from build123d import *

# Parameters (mm, degrees)
BOSS_EXTRUDE1_DEPTH = 10
FILLET1_R           = 1
FILLET2_R           = 0.5
FILLET3_R           = 1


with BuildPart() as part:
    # Sketch1 → Boss-Extrude1 (new body)
    with BuildSketch(Plane.XY):
        with BuildLine():
            Line((0.05, 14.37), (0.05, 3.706076092))
            ThreePointArc((0.05, 3.706076092), (1.009905384, 4.156578123), (2.05, 4.362911872))
            Line((2.05, 4.362911872), (2.05, 14.37))
            ThreePointArc((2.05, 14.37), (0.989726548, 16.929726548), (-1.57, 17.99))
            Line((-1.57, 17.99), (-2.748, 17.99))
            ThreePointArc((-2.748, 17.99), (-5.307726548, 16.929726548), (-6.368, 14.37))
            Line((-6.368, 14.37), (-4.368, 14.37))
            ThreePointArc((-4.368, 14.37), (-3.893512986, 15.515512986), (-2.748, 15.99))
            Line((-2.748, 15.99), (-1.57, 15.99))
            ThreePointArc((-1.57, 15.99), (-0.424487014, 15.515512986), (0.05, 14.37))
        make_face()
        with BuildLine():
            Line((0.05, -0.484767986), (0.05, -3.706076092))
            ThreePointArc((0.05, -3.706076092), (1.009905384, -4.156578123), (2.05, -4.362911872))
            Line((2.05, -4.362911872), (2.05, -2.352658071))
            ThreePointArc((2.05, -2.352658071), (0.753926793, -1.73572655), (0.05, -0.484767986))
        make_face()
        with BuildLine():
            ThreePointArc((2.05, 4.362911872), (1.009905384, 4.156578123), (0.05, 3.706076092))
            Line((0.05, 3.706076092), (0.05, 0.484767986))
            ThreePointArc((0.05, 0.484767986), (0.753926793, 1.73572655), (2.05, 2.352658071))
            Line((2.05, 2.352658071), (2.05, 4.362911872))
        make_face()
        with BuildLine():
            Line((2.05, -2.352658071), (2.05, -4.362911872))
            ThreePointArc((2.05, -4.362911872), (5.351470225, -3.206438835), (6.75, 0))
            ThreePointArc((6.75, 0), (5.351470225, 3.206438835), (2.05, 4.362911872))
            Line((2.05, 4.362911872), (2.05, 2.352658071))
            ThreePointArc((2.05, 2.352658071), (3.935248378, 1.790600458), (4.75, 0))
            ThreePointArc((4.75, 0), (3.935248378, -1.790600458), (2.05, -2.352658071))
        make_face()
        with BuildLine():
            Line((-1.57, -15.99), (-2.748, -15.99))
            ThreePointArc((-2.748, -15.99), (-3.893512986, -15.515512986), (-4.368, -14.37))
            Line((-4.368, -14.37), (-6.368, -14.37))
            ThreePointArc((-6.368, -14.37), (-5.307726548, -16.929726548), (-2.748, -17.99))
            Line((-2.748, -17.99), (-1.57, -17.99))
            ThreePointArc((-1.57, -17.99), (0.989726548, -16.929726548), (2.05, -14.37))
            Line((2.05, -14.37), (2.05, -4.362911872))
            ThreePointArc((2.05, -4.362911872), (1.009905384, -4.156578123), (0.05, -3.706076092))
            Line((0.05, -3.706076092), (0.05, -14.37))
            ThreePointArc((0.05, -14.37), (-0.424487014, -15.515512986), (-1.57, -15.99))
        make_face()
    extrude(amount=BOSS_EXTRUDE1_DEPTH)

    # Fillet1
    fillet1_edges = [part.edges().sort_by_distance(p)[0] for p in [
        (0.05, -0.484767986, 5),
        (0.05, 0.484767986, 5),
    ]]
    fillet(fillet1_edges, radius=FILLET1_R)

    # Fillet2
    fillet2_edges = [part.edges().sort_by_distance(p)[0] for p in [
        (2.05, 4.362911872, 5),
        (2.05, -4.362911872, 5),
    ]]
    fillet(fillet2_edges, radius=FILLET2_R)

    # Fillet3
    fillet3_edges = [part.edges().sort_by_distance(p)[0] for p in [
        (-6.368, 14.37, 5),
        (-4.368, 14.37, 5),
        (-6.368, -14.37, 5),
        (-4.368, -14.37, 5),
    ]]
    fillet(fillet3_edges, radius=FILLET3_R - 0.0001)  # a hair under: the kernel refuses the full size


solid = part.part
For this review, take the finished solid that the model builds, in its own axes (mm). A direction names the side the tool comes from. Give positions to 0.01 mm unless a question says otherwise; leave off trailing zeros. Loops run counter-clockwise (first coordinate to the right, second up) from the corner with the lowest first, then second, coordinate; pieces in that order, holes last.
Item 1: Take a section at D-D, the plane x = 6. State the section outline as (y, z) points, and give its area (3 significant figures).
Item 2: Draft analysis for pull direction Y (two halves, no side actions). For faces 5 (the flat face through (1, 3, 0)), 6 (the cylindrical face through (0.51, -2.26, 5.07)), 7 (the cylindrical face through (1.02, 16.9, 4.93)), 8 (the cylindrical face through (0.96, -16.96, 4.93)), state which applies: +Y half, -Y half, draft (parallel to the pull), parting line (faces both ways), or undercut.
Item 3: Take a section at C-C, the plane y = -1.5. State the section outline as (x, z) points, and give its area (3 significant figures).
Item 4: Tool access review of faces 1 (the flat face through (0.05, 9, 5)), 2 (the flat face through (2.05, -10, 5)), 3 (the flat face through (-2, -15.99, 5)), 4 (the flat face through (2.05, 10, 5)): name each direction out of +Z, -Z, +X, -X, +Y, -Y from which nothing blocks a thin tool from reaching the whole face with its end or side.
Item 5: For line 1 along Y through (x, z) = (-2.5, 9.25); line 2 along X through (y, z) = (-10, 7.75); line 3 along Y through (x, z) = (4, 1.75), list the stretches that pass through material, from the lowest coordinate up.
Item 6: Take a section at A-A, the plane x = -1.25. State the section outline as (y, z) points.
Item 7: Insertion check: pin 1 (1.5 mm diameter, centred on y = -1.5, z = 2.5, fed in from +X); pin 2 (3 mm diameter, centred on y = -9, z = 3.5, fed in from +X); pin 3 (5 mm diameter, centred on y = 2, z = 4, fed in from -X); pin 4 (2 mm diameter, centred on x = 4, y = 5.5, fed in from -Z). Each pin has a flat end and moves straight along its axis. Give the tip position at first contact, or say it passes through.
Calculated:
1. outline: (-2.45, 0) - (2.45, 0) - (2.45, 10) - (-2.45, 10) - close
1. area: 49.0 mm2
2. face 5: draft
2. face 6: undercut
2. face 7: +Y half
2. face 8: -Y half
3. outline: (4.22, 0) - (6.48, 0) - (6.48, 10) - (4.22, 10) - close
3. area: 22.7 mm2
4. face 1: +Z, -Z, -X
4. face 2: +Z, -Z, +X, -Y
4. face 3: +Z, -Z
4. face 4: +Z, -Z, +X, +Y
5. line 1: y = -17.99 to -15.99, 15.99 to 17.99
5. line 2: x = 0.05 to 2.05
5. line 3: y = -4.06 to -1.73, 1.73 to 4.06
6. outline: (-17.98, 0) - (-15.96, 0) - (-15.96, 10) - (-17.98, 10) - close; (15.96, 0) - (17.98, 0) - (17.98, 10) - (15.96, 10) - close
7. pin 1: stops at x = 6.69
7. pin 2: stops at x = 2.05
7. pin 3: stops at x = 0.05
7. pin 4: passes through
